Verification items for the finished model (mm, model axes). Face numbers are marked on the shaded views. A direction names the side the tool comes from. Give positions to 0.01 mm unless a question says otherwise; leave off trailing zeros. Write each loop counter-clockwise with the first axis right and the second up, starting at its lowest first coordinate (ties: lowest second). Pieces come first, ordered by that corner, then holes. Notation, with made-up numbers: (-14.5, 63.5) - (31.5, 63.5) arc R3 ccw to (31.5, 68.5) - close; hole circle Ø3 at (32.5, 25). An arc over 180 degrees is marked (long way). Answer as a JSON object with one key per item and string values. Group by question number.
Item 1: Sectioned sample at C-C, the plane x = -5. Record the boundary of the cut face in (y, z), and give its area (3 significant figures).
Item 2: Sectioned sample at A-A, the plane y = -3.5. Record the boundary of the cut face in (x, z).
Item 3: Sectioned sample at D-D, the plane y = -12.5. Record the boundary of the cut face in (x, z).
Item 4: Tool access check on the marked faces 4 and 5. Record the directions out of +Z, -Z, +X, -X, +Y, -Y that give a thin tool (end or side, any length) a straight path to the whole face; none if there is none.
Item 5: Go/stop test with flat-tipped pins: pin 1 (8 mm diameter, centred on x = 38.5, y = -17, fed in from +Z); pin 2 (1.9 mm diameter, centred on x = 5, z = -14.5, fed in from +Y); pin 3 (4 mm diameter, centred on y = -32.5, z = 16, fed in from +X); pin 4 (2 mm diameter, centred on x = 24, y = -27, fed in from -Z). Record where each tip stops, or that it passes through.
Item 6: Scan lines: line 1 along Z through (x, y) = (-5, -32); line 2 along Z through (x, y) = (-50, -6.75); line 3 along X through (y, z) = (-31, 19). Record each from-to range of solid material in increasing order. Write a range as [from, to].
Item 7: Draft check along X on the marked faces 1, 2 and 3. Enter one of: +X half, -X half, draft (parallel to the pull), parting line (faces both ways), or undercut.
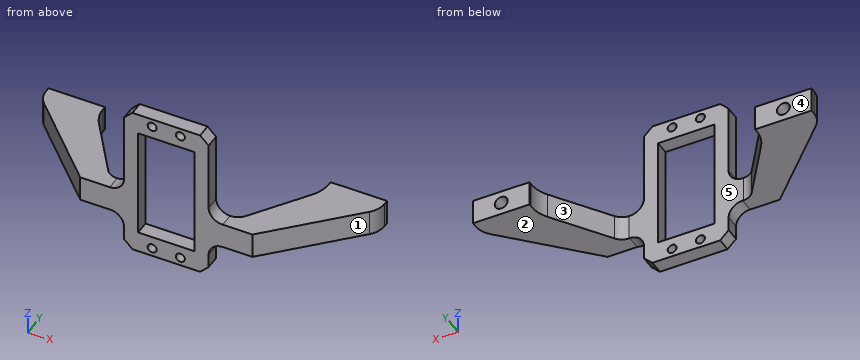
```python
from build123d import *

# Parameters (mm, degrees)
PAD005_DEPTH    = 4.5
SKETCH013_R     = 2.3
POCKET009_DEPTH = 10
SKETCH014_W     = 30
SKETCH014_H     = 55
SKETCH014_R     = 1.6
SKETCH014_W_2   = 20
SKETCH014_H_2   = 40
PAD006_DEPTH    = 5
FILLET007_R     = 12
FILLET008_R     = 5
FILLET009_R     = 8
CHAMFER009_SIZE = 3
FILLET010_R     = 5


with BuildPart() as part:
    # Sketch012 → Pad005 (new body, symmetric)
    with BuildSketch(Plane.XY):
        Polygon((-60, 0), (-60, -5), (-30.5, -34.5), (-10, -34.5), (-10, -29.5), (-22.844915, -29.5), (-40, -5), (-40, 0), align=None)
    pad005 = extrude(amount=PAD005_DEPTH, both=True)

    # Sketch013 (on Face8 of Pad005) → Pocket009 (cut)
    with BuildSketch(Plane(origin=(0, 0, 0), x_dir=(-1, 0, 0), z_dir=(0, 1, 0))):
        with Locations((50, 0)):
            Circle(SKETCH013_R)
    pocket009 = extrude(amount=-POCKET009_DEPTH, mode=Mode.SUBTRACT)

    # Mirrored001: Pad005, Pocket009 across YZ
    add(pad005.mirror(Plane.YZ))
    add(pocket009.mirror(Plane.YZ), mode=Mode.SUBTRACT)

    # Sketch014 (on Face10 of Mirrored001) → Pad006 (join)
    with BuildSketch(Plane(origin=(0, -29.5, 0), x_dir=(-1, 0, 0), z_dir=(0, 1, 0))):
        with Locations((0, 10)):
            Rectangle(SKETCH014_W, SKETCH014_H)
        with Locations((5, 34.5)):
            Circle(SKETCH014_R, mode=Mode.SUBTRACT)
        with Locations((-5, 34.5)):
            Circle(SKETCH014_R, mode=Mode.SUBTRACT)
        with Locations((5, -14.5)):
            Circle(SKETCH014_R, mode=Mode.SUBTRACT)
        with Locations((-5, -14.5)):
            Circle(SKETCH014_R, mode=Mode.SUBTRACT)
        with Locations((0, 10)):
            Rectangle(SKETCH014_W_2, SKETCH014_H_2, mode=Mode.SUBTRACT)
    extrude(amount=-PAD006_DEPTH)

    # Fillet007
    fillet007_edges = [part.edges().sort_by_distance(p)[0] for p in [
        (-40, -5, 0),
        (40, -5, 0),
    ]]
    fillet(fillet007_edges, radius=FILLET007_R)

    # Fillet008
    fillet008_edges = [part.edges().sort_by_distance(p)[0] for p in [
        (22.844915, -29.5, 0),
        (-22.844915, -29.5, 0),
    ]]
    fillet(fillet008_edges, radius=FILLET008_R)

    # Fillet009
    fillet009_edges = [part.edges().sort_by_distance(p)[0] for p in [
        (60, -5, 0),
        (-60, -5, 0),
    ]]
    fillet(fillet009_edges, radius=FILLET009_R)

    # Chamfer009
    chamfer009_edges = [part.edges().sort_by_distance(p)[0] for p in [
        (15, -32, -17.5),
        (-15, -32, -17.5),
        (15, -32, 37.5),
        (-15, -32, 37.5),
    ]]
    chamfer(chamfer009_edges, length=CHAMFER009_SIZE)

    # Fillet010
    fillet010_edges = [part.edges().sort_by_distance(p)[0] for p in [
        (15, -32, 4.5),
        (15, -32, -4.5),
        (-15, -32, 4.5),
        (-15, -32, -4.5),
    ]]
    fillet(fillet010_edges, radius=FILLET010_R)


solid = part.part
```
Geometry check:
{
 "1": {"outline": "(-34.5, -17.5) - (-29.5, -17.5) - (-29.5, -16.1) - (-34.5, -16.1) - close; (-34.5, -12.9) - (-29.5, -12.9) - (-29.5, -10) - (-34.5, -10) - close; (-34.5, 30) - (-29.5, 30) - (-29.5, 32.9) - (-34.5, 32.9) - close; (-34.5, 36.1) - (-29.5, 36.1) - (-29.5, 37.5) - (-34.5, 37.5) - close", "area": "43.0 mm^2"},
 "2": {"outline": "(-59.79, -4.5) - (-39.78, -4.5) - (-39.78, 4.5) - (-59.79, 4.5) - close; (39.78, -4.5) - (59.79, -4.5) - (59.79, 4.5) - (39.78, 4.5) - close; hole circle Ø4.6 at (-50, 0); hole circle Ø4.6 at (50, 0)"},
 "3": {"outline": "(-52.5, -4.5) - (-34.75, -4.5) - (-34.75, 4.5) - (-52.5, 4.5) - close; (34.75, -4.5) - (52.5, -4.5) - (52.5, 4.5) - (34.75, 4.5) - close"},
 "4": {"face 4": "+Z, -Z, +X, -X, +Y", "face 5": "+Z, -Z, +Y"},
 "5": {"pin 1": "z = 4.5", "pin 2": "through", "pin 3": "x = 15", "pin 4": "z = -4.5"},
 "6": {"line 1": "[-17.5, -16.1], [-12.9, -10], [30, 32.9], [36.1, 37.5]", "line 2": "[-4.5, -2.3], [2.3, 4.5]", "line 3": "[-15, -10], [10, 15]"},
 "7": {"face 1": "+X half", "face 2": "draft", "face 3": "undercut"}
}
